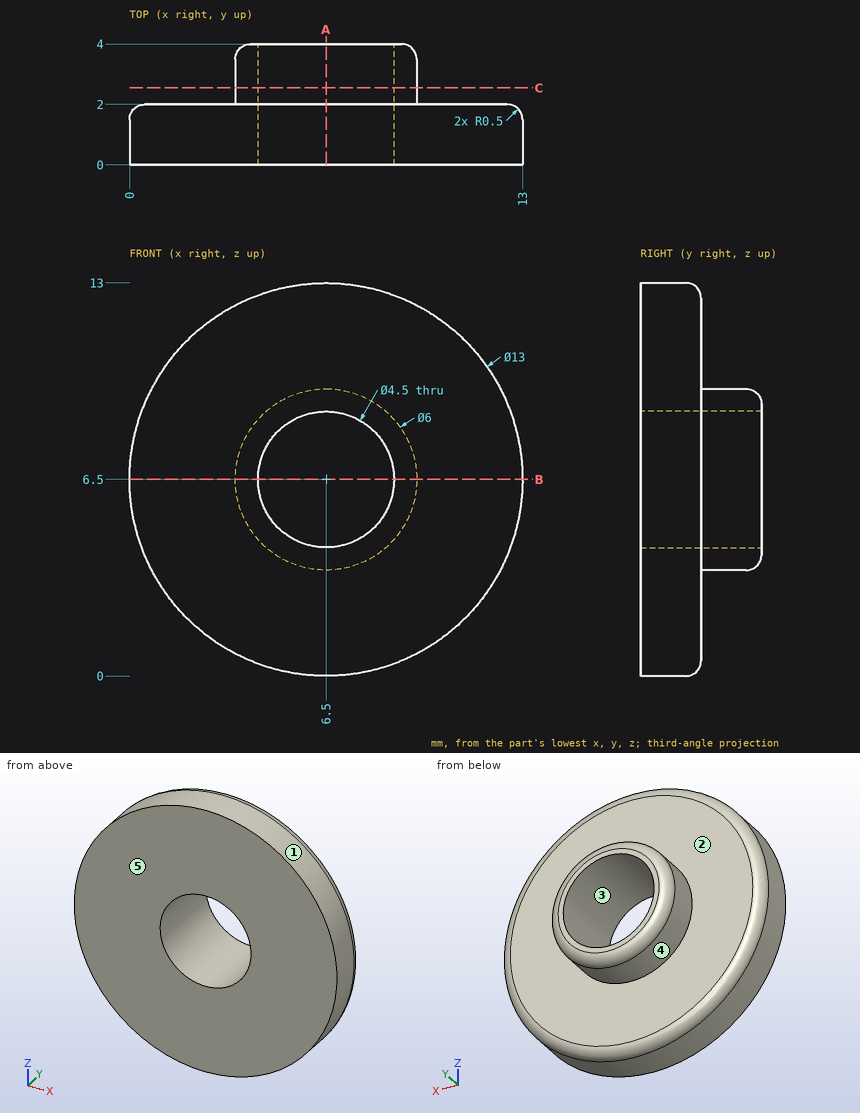
Source: three-view drawing plus pictorial views. Frame: mm from the lowest corner of the part. A direction names the side the tool comes from. Round coordinates to 2 decimals unless told otherwise and drop trailing zeros. Loops run counter-clockwise (first coordinate to the right, second up) from the corner with the lowest first, then second, coordinate; pieces in that order, holes last.
Item 1: Contact query for flat-ended pins moving along their axis: P1, Ø2, axis at x = 2.5, z = 6, coming from the +Y side; P2, Ø2, axis at x = 2, y = 2.5, coming from the -Z side. Output: stop coordinate, or through.
Checked values:
P1: stops at y = 2
P2: stops at z = 1.34
Item 2: Reachability of the marked faces 4 and 5 from +Z, -Z, +X, -X, +Y, -Y: full face, straight path, thin tool, end or side. Return the list, or none.
Checked values:
face 4: +Y
face 5: +Z, -Z, +X, -X, -Y
Item 3: Section C-C, the plane y = 2.55. Output: boundary loops of the cut face in (x, z), plus the area to 3 significant figures.
Checked values:
outline: circle Ø6 at (6.5, 6.5); hole circle Ø4.5 at (6.5, 6.5)
area: 12.4 mm2
Item 4: Mould query, pull axis Z, two halves, no side actions, for the marked faces 1, 2 and 3. Classes: released by +Z, released by -Z, zero draft, split by the parting line, or undercut.
Checked values:
face 1: split by the parting line
face 2: zero draft
face 3: undercut
Item 5: Section A-A, the plane x = 6.5. Output: boundary loops of the cut face in (y, z).
Checked values:
outline: (0, 0) - (1.5, 0) arc R0.5 ccw to (2, 0.5) - (2, 3.5) - (3.5, 3.5) arc R0.5 ccw to (4, 4) - (4, 4.25) - (0, 4.25) - close; (0, 8.75) - (4, 8.75) - (4, 9) arc R0.5 ccw to (3.5, 9.5) - (2, 9.5) - (2, 12.5) arc R0.5 ccw to (1.5, 13) - (0, 13) - close
Item 6: Section B-B, the plane z = 6.5. Output: boundary loops of the cut face in (x, y).
Checked values:
outline: (0, 0) - (4.25, 0) - (4.25, 4) - (4, 4) arc R0.5 ccw to (3.5, 3.5) - (3.5, 2) - (0.5, 2) arc R0.5 ccw to (0, 1.5) - close; (8.75, 0) - (13, 0) - (13, 1.5) arc R0.5 ccw to (12.5, 2) - (9.5, 2) - (9.5, 3.5) arc R0.5 ccw to (9, 4) - (8.75, 4) - close
Item 7: Line query: L1, parallel to X at y = 2.7, z = 6.5; L2, parallel to X at y = 1.15, z = 6.5; L3, parallel to Y at x = 12, z = 4.75. Output: solid intervals per line, ascending.
Checked values:
L1: x = 3.5 to 4.25, 8.75 to 9.5
L2: x = 0 to 4.25, 8.75 to 13
L3: y = 0 to 2
